from build123d import *

# Parameters (mm, degrees)
SKETCH_1_R      = 1.6
SKETCH_1_R_2    = 5
SKETCH_1_R_3    = 1.5
EXTRUDE_1_DEPTH = 4


with BuildPart() as part:
    # 草图1 → 凸台-拉伸1 (new body)
    with BuildSketch(Plane.XY):
        with BuildLine():
            Line((-16.419786686, 79.176264565), (-1.041261143, 72.941727182))
            Line((-1.041261143, 72.941727182), (-1.041261143, 12.941727182))
            ThreePointArc((-1.041261143, 12.941727182), (1.887671046, 5.87065937), (8.958738857, 2.941727182))
            Line((8.958738857, 2.941727182), (86.958738857, 2.941727182))
            ThreePointArc((86.958738857, 2.941727182), (94.029806669, 5.87065937), (96.958738857, 12.941727182))
            Line((96.958738857, 12.941727182), (96.958738857, 72.941727182))
            Line((96.958738857, 72.941727182), (112.337264401, 79.176264565))
            ThreePointArc((112.337264401, 79.176264565), (114.605582701, 81.01645305), (115.458738857, 83.809960906))
            Line((115.458738857, 83.809960906), (115.458738857, 102.073493459))
            ThreePointArc((115.458738857, 102.073493459), (114.605582701, 104.867001314), (112.337264401, 106.7071898))
            Line((112.337264401, 106.7071898), (96.958738857, 112.941727182))
            Line((96.958738857, 112.941727182), (96.958738857, 177.941727182))
            ThreePointArc((96.958738857, 177.941727182), (95.494272763, 181.477261088), (91.958738857, 182.941727182))
            Line((91.958738857, 182.941727182), (3.958738857, 182.941727182))
            ThreePointArc((3.958738857, 182.941727182), (0.423204952, 181.477261088), (-1.041261143, 177.941727182))
            Line((-1.041261143, 177.941727182), (-1.041261143, 112.941727182))
            Line((-1.041261143, 112.941727182), (-16.419786686, 106.7071898))
            ThreePointArc((-16.419786686, 106.7071898), (-18.688104986, 104.867001314), (-19.541261143, 102.073493459))
            Line((-19.541261143, 102.073493459), (-19.541261143, 83.809960906))
            ThreePointArc((-19.541261143, 83.809960906), (-18.688104986, 81.01645305), (-16.419786686, 79.176264565))
        make_face()
        with Locations((22.958738857, 161.441727182)):
            Circle(SKETCH_1_R, mode=Mode.SUBTRACT)
        with Locations((72.958738857, 145.441727182)):
            Circle(SKETCH_1_R, mode=Mode.SUBTRACT)
        with Locations((72.958738857, 24.441727182)):
            Circle(SKETCH_1_R, mode=Mode.SUBTRACT)
        with Locations((72.958738857, 40.441727182)):
            Circle(SKETCH_1_R, mode=Mode.SUBTRACT)
        with Locations((86.958738857, 40.441727182)):
            Circle(SKETCH_1_R, mode=Mode.SUBTRACT)
        with Locations((86.958738857, 145.441727182)):
            Circle(SKETCH_1_R, mode=Mode.SUBTRACT)
        with Locations((86.958738857, 161.441727182)):
            Circle(SKETCH_1_R, mode=Mode.SUBTRACT)
        with Locations((72.958738857, 161.441727182)):
            Circle(SKETCH_1_R, mode=Mode.SUBTRACT)
        with Locations((22.958738857, 40.441727182)):
            Circle(SKETCH_1_R, mode=Mode.SUBTRACT)
        with Locations((8.958738857, 145.441727182)):
            Circle(SKETCH_1_R, mode=Mode.SUBTRACT)
        with Locations((8.958738857, 161.441727182)):
            Circle(SKETCH_1_R, mode=Mode.SUBTRACT)
        with Locations((22.958738857, 145.441727182)):
            Circle(SKETCH_1_R, mode=Mode.SUBTRACT)
        with Locations((86.958738857, 24.441727182)):
            Circle(SKETCH_1_R, mode=Mode.SUBTRACT)
        with Locations((8.958738857, 24.441727182)):
            Circle(SKETCH_1_R, mode=Mode.SUBTRACT)
        with Locations((8.958738857, 40.441727182)):
            Circle(SKETCH_1_R, mode=Mode.SUBTRACT)
        with Locations((22.958738857, 24.441727182)):
            Circle(SKETCH_1_R, mode=Mode.SUBTRACT)
        with Locations((40.958738857, 174.941727182)):
            Circle(SKETCH_1_R, mode=Mode.SUBTRACT)
        with Locations((75.958738857, 140.941727182)):
            Circle(SKETCH_1_R, mode=Mode.SUBTRACT)
        with Locations((54.958738857, 174.941727182)):
            Circle(SKETCH_1_R, mode=Mode.SUBTRACT)
        with Locations((19.958738857, 52.941727182)):
            Circle(SKETCH_1_R, mode=Mode.SUBTRACT)
        with Locations((19.958738857, 44.941727182)):
            Circle(SKETCH_1_R, mode=Mode.SUBTRACT)
        with Locations((75.958738857, 44.941727182)):
            Circle(SKETCH_1_R, mode=Mode.SUBTRACT)
        with Locations((75.958738857, 132.941727182)):
            Circle(SKETCH_1_R, mode=Mode.SUBTRACT)
        with Locations((19.958738857, 132.941727182)):
            Circle(SKETCH_1_R, mode=Mode.SUBTRACT)
        with Locations((19.958738857, 140.941727182)):
            Circle(SKETCH_1_R, mode=Mode.SUBTRACT)
        with Locations((75.958738857, 52.941727182)):
            Circle(SKETCH_1_R, mode=Mode.SUBTRACT)
        with Locations((35.958738857, 136.941727182)):
            Circle(SKETCH_1_R, mode=Mode.SUBTRACT)
        with Locations((97.458738857, 82.941727182)):
            Circle(SKETCH_1_R, mode=Mode.SUBTRACT)
        with Locations((105.458738857, 82.941727182)):
            Circle(SKETCH_1_R, mode=Mode.SUBTRACT)
        with Locations((97.458738857, 92.941727182)):
            Circle(SKETCH_1_R, mode=Mode.SUBTRACT)
        with Locations((105.458738857, 92.941727182)):
            Circle(SKETCH_1_R, mode=Mode.SUBTRACT)
        with Locations((-9.541261143, 82.941727182)):
            Circle(SKETCH_1_R, mode=Mode.SUBTRACT)
        with Locations((-1.541261143, 82.941727182)):
            Circle(SKETCH_1_R, mode=Mode.SUBTRACT)
        with Locations((-1.541261143, 92.941727182)):
            Circle(SKETCH_1_R, mode=Mode.SUBTRACT)
        with Locations((-9.541261143, 92.941727182)):
            Circle(SKETCH_1_R, mode=Mode.SUBTRACT)
        with Locations((-1.541261143, 102.941727182)):
            Circle(SKETCH_1_R, mode=Mode.SUBTRACT)
        with Locations((-9.541261143, 102.941727182)):
            Circle(SKETCH_1_R, mode=Mode.SUBTRACT)
        with Locations((83.958738857, 136.941727182)):
            Circle(SKETCH_1_R, mode=Mode.SUBTRACT)
        with Locations((59.958738857, 136.941727182)):
            Circle(SKETCH_1_R, mode=Mode.SUBTRACT)
        with Locations((59.958738857, 166.941727182)):
            Circle(SKETCH_1_R, mode=Mode.SUBTRACT)
        with Locations((15.958738857, 117.941727182)):
            Circle(SKETCH_1_R, mode=Mode.SUBTRACT)
        with Locations((35.958738857, 166.941727182)):
            Circle(SKETCH_1_R, mode=Mode.SUBTRACT)
        with Locations((11.958738857, 136.941727182)):
            Circle(SKETCH_1_R, mode=Mode.SUBTRACT)
        with Locations((11.958738857, 166.941727182)):
            Circle(SKETCH_1_R, mode=Mode.SUBTRACT)
        with Locations((83.958738857, 166.941727182)):
            Circle(SKETCH_1_R, mode=Mode.SUBTRACT)
        with Locations((105.458738857, 102.941727182)):
            Circle(SKETCH_1_R, mode=Mode.SUBTRACT)
        with Locations((97.458738857, 102.941727182)):
            Circle(SKETCH_1_R, mode=Mode.SUBTRACT)
        with Locations((47.958738857, 92.941727182)):
            Circle(SKETCH_1_R_2, mode=Mode.SUBTRACT)
        with Locations((79.958738857, 117.941727182)):
            Circle(SKETCH_1_R, mode=Mode.SUBTRACT)
        with Locations((79.958738857, 59.941727182)):
            Circle(SKETCH_1_R, mode=Mode.SUBTRACT)
        with Locations((15.958738857, 59.941727182)):
            Circle(SKETCH_1_R, mode=Mode.SUBTRACT)
        with Locations((77.958738857, 175.441727182)):
            Circle(SKETCH_1_R, mode=Mode.SUBTRACT)
        with Locations((17.958738857, 175.441727182)):
            Circle(SKETCH_1_R, mode=Mode.SUBTRACT)
        with Locations((17.958738857, 10.441727182)):
            Circle(SKETCH_1_R, mode=Mode.SUBTRACT)
        with Locations((77.958738857, 10.441727182)):
            Circle(SKETCH_1_R, mode=Mode.SUBTRACT)
        with Locations((26.246162591, 107.185151506)):
            Circle(SKETCH_1_R_3, mode=Mode.SUBTRACT)
        with Locations((26.246162591, 63.185151506)):
            Circle(SKETCH_1_R_3, mode=Mode.SUBTRACT)
        with Locations((70.246162591, 63.185151506)):
            Circle(SKETCH_1_R_3, mode=Mode.SUBTRACT)
        with Locations((70.246162591, 107.185151506)):
            Circle(SKETCH_1_R_3, mode=Mode.SUBTRACT)
        with Locations((47.960174004, 166.120088822)):
            Circle(SKETCH_1_R_3, mode=Mode.SUBTRACT)
        with Locations((47.960174004, 150.120088822)):
            Circle(SKETCH_1_R_3, mode=Mode.SUBTRACT)
        with Locations((39.960174004, 158.120088822)):
            Circle(SKETCH_1_R_3, mode=Mode.SUBTRACT)
        with Locations((55.960174004, 158.120088822)):
            Circle(SKETCH_1_R_3, mode=Mode.SUBTRACT)
        with Locations((47.960174004, 159.79228367)):
            Circle(SKETCH_1_R_3, mode=Mode.SUBTRACT)
        with Locations((47.960174004, 143.79228367)):
            Circle(SKETCH_1_R_3, mode=Mode.SUBTRACT)
        with Locations((47.960174004, 155.046429946)):
            Circle(SKETCH_1_R_3, mode=Mode.SUBTRACT)
        with Locations((47.960174004, 139.046429946)):
            Circle(SKETCH_1_R_3, mode=Mode.SUBTRACT)
        with BuildLine():
            Line((71.958738857, 87.941727182), (71.958738857, 97.941727182))
            ThreePointArc((71.958738857, 97.941727182), (67.958738857, 101.941727182), (63.958738857, 97.941727182))
            Line((63.958738857, 97.941727182), (63.958738857, 87.941727182))
            ThreePointArc((63.958738857, 87.941727182), (67.958738857, 83.941727182), (71.958738857, 87.941727182))
        make_face(mode=Mode.SUBTRACT)
        with BuildLine():
            Line((31.958738857, 87.941727182), (31.958738857, 97.941727182))
            ThreePointArc((31.958738857, 97.941727182), (27.958738857, 101.941727182), (23.958738857, 97.941727182))
            Line((23.958738857, 97.941727182), (23.958738857, 87.941727182))
            ThreePointArc((23.958738857, 87.941727182), (27.958738857, 83.941727182), (31.958738857, 87.941727182))
        make_face(mode=Mode.SUBTRACT)
        with BuildLine():
            Line((61.063788273, 106.79385107), (72.178592544, 116.866642441))
            ThreePointArc((72.178592544, 116.866642441), (72.282793834, 118.985402005), (70.16403427, 119.089603295))
            Line((70.16403427, 119.089603295), (59.049229998, 109.016811924))
            ThreePointArc((59.049229998, 109.016811924), (58.945028708, 106.89805236), (61.063788273, 106.79385107))
        make_face(mode=Mode.SUBTRACT)
        with BuildLine():
            Line((36.868247717, 109.016811924), (25.753443445, 119.089603295))
            ThreePointArc((25.753443445, 119.089603295), (23.634683881, 118.985402005), (23.738885171, 116.866642441))
            Line((23.738885171, 116.866642441), (34.853689442, 106.79385107))
            ThreePointArc((34.853689442, 106.79385107), (36.972449007, 106.89805236), (36.868247717, 109.016811924))
        make_face(mode=Mode.SUBTRACT)
        with BuildLine():
            Line((34.853689442, 79.089603295), (23.738885171, 69.016811924))
            ThreePointArc((23.738885171, 69.016811924), (23.634683881, 66.89805236), (25.753443445, 66.79385107))
            Line((25.753443445, 66.79385107), (36.868247717, 76.866642441))
            ThreePointArc((36.868247717, 76.866642441), (36.972449007, 78.985402005), (34.853689442, 79.089603295))
        make_face(mode=Mode.SUBTRACT)
        with BuildLine():
            Line((59.049229998, 76.866642441), (70.16403427, 66.79385107))
            ThreePointArc((70.16403427, 66.79385107), (72.282793834, 66.89805236), (72.178592544, 69.016811924))
            Line((72.178592544, 69.016811924), (61.063788273, 79.089603295))
            ThreePointArc((61.063788273, 79.089603295), (58.945028708, 78.985402005), (59.049229998, 76.866642441))
        make_face(mode=Mode.SUBTRACT)
        with BuildLine():
            Line((32.958738857, 43.441727182), (62.958738857, 43.441727182))
            ThreePointArc((62.958738857, 43.441727182), (64.458738857, 44.941727182), (62.958738857, 46.441727182))
            Line((62.958738857, 46.441727182), (32.958738857, 46.441727182))
            ThreePointArc((32.958738857, 46.441727182), (31.458738857, 44.941727182), (32.958738857, 43.441727182))
        make_face(mode=Mode.SUBTRACT)
        with BuildLine():
            Line((32.958738857, 13.441727182), (62.958738857, 13.441727182))
            ThreePointArc((62.958738857, 13.441727182), (64.458738857, 14.941727182), (62.958738857, 16.441727182))
            Line((62.958738857, 16.441727182), (32.958738857, 16.441727182))
            ThreePointArc((32.958738857, 16.441727182), (31.458738857, 14.941727182), (32.958738857, 13.441727182))
        make_face(mode=Mode.SUBTRACT)
    extrude(amount=EXTRUDE_1_DEPTH)


solid = part.part
Geometry check sheet. Reference: the model listing, model coordinates, mm. A direction names the side the tool comes from. Round coordinates to 2 decimals unless told otherwise and drop trailing zeros. One line per question, with ' | ' between items. Start each with the question number.
1. Tool access check on faces 1 (the face through (48, 43.442, 2)), 2 (the face through (-1.041, 146, 2)), 3 (the face through (115.459, 93, 2)). Record the directions out of +Z, -Z, +X, -X, +Y, -Y that give a thin tool (end or side, any length) a straight path to the whole face; none if there is none.
2. Scan lines: line 1 (Y direction, x = 25.5, z = 3.7); line 2 (Y direction, x = 50, z = 2); line 3 (X direction, y = 155, z = 0.75). Record each from-to range of solid material in increasing order. Write a range as [from, to].
3. Cross-section at A-A on z = 2.75. State how many separate pieces and enclosed holes the cut face has, then the cut area to 3 significant figures.
4. Depth check by flat-ended pin: pin 1 (1 mm diameter, centred on y = 47, z = 2.5, fed in from -X); pin 2 (1 mm diameter, centred on y = 74, z = 2.5, fed in from -X) (3 decimals). Enter the tip coordinate at first touch or a pass-through.
5. Draft check along X on faces 4 (the face through (48, 16.442, 2)), 5 (the face through (104.5, 76, 2)), 6 (the face through (-8.838, 76.103, 1.972)). Enter one of: released by +X, released by -X, zero draft, split by the parting line, or undercut.
Taken from the geometry:
1) face 1: +Z, -Z | face 2: +Z, -Z, -X, +Y | face 3: +Z, -Z, +X, +Y, -Y
2) line 1: [2.94, 61.88], [64.49, 66.61], [70.61, 84.79], [101.1, 105.88], [108.49, 115.27], [119.27, 182.94] | line 2: [2.94, 13.44], [16.44, 43.44], [46.44, 88.38], [97.51, 182.94] | line 3: [-1.04, 46.46], [49.46, 96.96]
3) separate pieces: 1 | enclosed holes: 75 | area: 17,500 mm²
4) pin 1: x = -1.04 | pin 2: x = -4.885
5) face 4: undercut | face 5: released by +X | face 6: released by -X
